Here's the drawing with two shaded views (mm, measured from the low corner). I have some questions. A direction names the side the tool comes from. Coordinates: 2 decimals unless noted, no trailing zeros. Loops run counter-clockwise (first coordinate to the right, second up) from the corner with the lowest first, then second, coordinate; pieces in that order, holes last. Notation, with made-up numbers: (-1, -11) -> (39, -11) arc R24 cw to (39, 27) -> close; hole circle Ø5 at (80, 79.25). An arc over 180 degrees is marked (long way). Use CSV: the item, a comma, the result in double quotes. Start each with the question number.
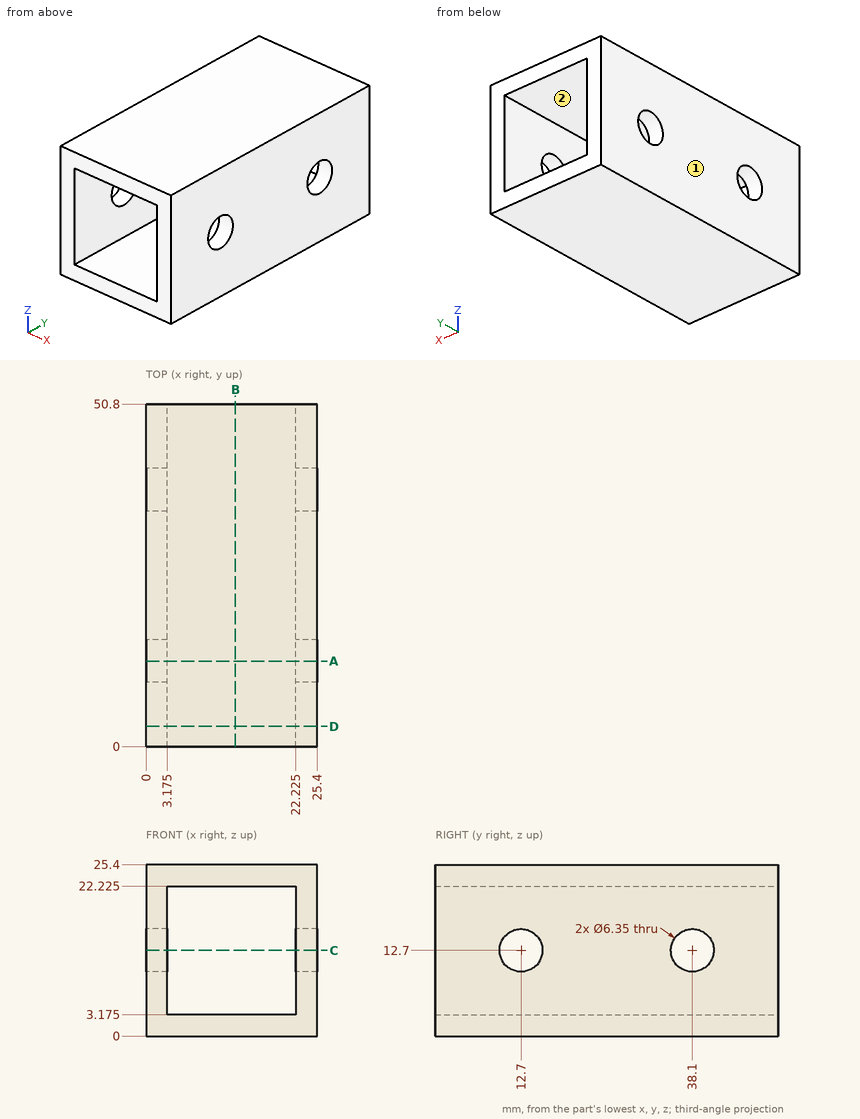
1) I want a section at B-B, the plane x = 13.25. Please give me the cut outline in (y, z) (3 decimals).
2) I want a section at C-C, the plane z = 12.7. Please give me the cut outline in (x, y) (3 decimals), plus the area to 3 significant figures.
3) Which directions (+Z, -Z, +X, -X, +Y, -Y) give clear straight access to the entire face, cutting with the end or side of a thin tool? Please do the marked faces 1 and 2.
4) I want a section at D-D, the plane y = 3. Please give me the cut outline in (x, z) (3 decimals).
5) I want a section at A-A, the plane y = 12.7. Please give me the cut outline in (x, z) (3 decimals).
6) Please list where these lines run through material, in increasing order: L1, parallel to Y at x = 2.5, z = 12.7 (3 decimals); L2, parallel to Z at x = 1.15, y = 38.1 (3 decimals); L3, parallel to Z at x = 20.5, y = 14 (3 decimals). Write a range as [from, to].
Return value:
1,outline,"(0, 0) -> (50.8, 0) -> (50.8, 3.175) -> (0, 3.175) -> close; (0, 22.225) -> (50.8, 22.225) -> (50.8, 25.4) -> (0, 25.4) -> close"
2,outline,"(0, 0) -> (3.175, 0) -> (3.175, 9.525) -> (0, 9.525) -> close; (0, 15.875) -> (3.175, 15.875) -> (3.175, 34.925) -> (0, 34.925) -> close; (0, 41.275) -> (3.175, 41.275) -> (3.175, 50.8) -> (0, 50.8) -> close; (22.225, 0) -> (25.4, 0) -> (25.4, 9.525) -> (22.225, 9.525) -> close; (22.225, 15.875) -> (25.4, 15.875) -> (25.4, 34.925) -> (22.225, 34.925) -> close; (22.225, 41.275) -> (25.4, 41.275) -> (25.4, 50.8) -> (22.225, 50.8) -> close"
2,area,"242 mm²"
3,face 1,"+Z, -Z, -X, +Y, -Y"
3,face 2,"+Y, -Y"
4,outline,"(0, 0) -> (25.4, 0) -> (25.4, 25.4) -> (0, 25.4) -> close; hole (3.175, 3.175) -> (22.225, 3.175) -> (22.225, 22.225) -> (3.175, 22.225) -> close"
5,outline,"(0, 0) -> (25.4, 0) -> (25.4, 9.525) -> (22.225, 9.525) -> (22.225, 3.175) -> (3.175, 3.175) -> (3.175, 9.525) -> (0, 9.525) -> close; (0, 15.875) -> (3.175, 15.875) -> (3.175, 22.225) -> (22.225, 22.225) -> (22.225, 15.875) -> (25.4, 15.875) -> (25.4, 25.4) -> (0, 25.4) -> close"
6,L1,"y = [0, 9.525], [15.875, 34.925], [41.275, 50.8]"
6,L2,"z = [0, 9.525], [15.875, 25.4]"
6,L3,"z = [0, 3.175], [22.225, 25.4]"
